Here's how the part is built. I have some questions about the finished solid (model axes, mm). Face numbers are marked on the shaded views. Give positions to 0.01 mm unless a question says otherwise; leave off trailing zeros. Write each loop counter-clockwise with the first axis right and the second up, starting at its lowest first coordinate (ties: lowest second). Pieces come first, ordered by that corner, then holes. Notation, with made-up numbers: (23, 53) - (48, 53) arc R26 cw to (48, 92) - close; hole circle Ø3 at (0.25, 10). An arc over 180 degrees is marked (long way). One line per item, written item: value. Start each with the question number.
1) Imagine slicing it at C-C on x = -8.5. Write out the boundary of the cut face in (y, z) (1 decimal), plus the area to 3 significant figures.
2) Imagine slicing it at D-D on z = -12.75. Write out the boundary of the cut face in (x, y).
3) Please list where these lines run through material, in increasing order: L1, parallel to Z at x = -2, y = -1; L2, parallel to Z at x = -9.75, y = -0.5 (1 decimal); L3, parallel to X at y = -1.1, z = -22. Write a range as [from, to].
4) We'd pull the mould along X, two halves only. Please class the marked faces 1 and 2: +X half, -X half, draft (parallel to the pull), parting line (faces both ways), or undercut.
5) Imagine slicing it at A-A on z = -18.5. Write out the boundary of the cut face in (x, y).
6) I'm going to push flat-ended pins straight in: P1, Ø0.8, axis at x = -8.5, y = -1.5, coming from the -Z side; P2, Ø5, axis at x = -7.5, z = -10, coming from the -Y side. Where does each tip first touch, or does it pass through?
Autodesk Inventor part; units mm, degrees
ref_plane "YZ Plane" through (0, 0, 0) normal (1, 0, 0) x (0, 1, 0)
ref_plane "XZ Plane" through (0, 0, 0) normal (0, 1, 0) x (-1, 0, 0)
ref_plane "XY Plane" through (0, 0, 0) normal (0, 0, 1) x (1, 0, 0)
sketch "Sketch1" plane through (0, 0, 0) normal (0, 1, 0) x (-1, 0, 0)
  line L0 (0, 0) -> (19.05, 0)
  line L1 (19.05, 0) -> (19.05, -24.003)
  line L2 (19.05, -24.003) -> (0, -24.003)
  line L3 (0, -24.003) -> (0, 0)
  dimension "d0" = 24.003
  dimension "d1" = 19.05
extrude "Extrusion1" add sketch "Sketch1" against normal blind 0.7937
fillet "Fillet1" radius 0.508 4 edges at (0, -0.3969, 0) (-19.05, -0.3969, 0) (0, -0.3969, -24.003) (-19.05, -0.3969, -24.003)
sketch "Sketch2" plane through (0, -0.7937, 0) normal (0, -1, 0) x (1, 0, 0)
  line L0 (-18.542, -24.003) -> (-0.508, -24.003)
  line L1 (0, -23.495) -> (0, -0.508)
  line L2 (-0.508, 0) -> (-18.542, 0)
  line L3 (-19.05, -0.508) -> (-19.05, -23.495)
  line L4 (-0.4572, -0.4572) -> (-18.5928, -0.4572)
  line L5 (-18.5928, -0.4572) -> (-18.5928, -23.5458)
  line L6 (-18.5928, -23.5458) -> (-0.4572, -23.5458)
  line L7 (-0.4572, -23.5458) -> (-0.4572, -0.4572)
  line L8 (-1.143, -1.143) -> (-17.907, -1.143)
  line L9 (-17.907, -1.143) -> (-17.907, -22.86)
  line L10 (-17.907, -22.86) -> (-1.143, -22.86)
  line L11 (-1.143, -22.86) -> (-1.143, -1.143)
  arc A0 (-19.05, -23.495) -> (-18.542, -24.003) centre (-18.542, -23.495) ccw
  arc A1 (-0.508, -24.003) -> (0, -23.495) centre (-0.508, -23.495) ccw
  arc A2 (0, -0.508) -> (-0.508, 0) centre (-0.508, -0.508) ccw
  arc A3 (-18.542, 0) -> (-19.05, -0.508) centre (-18.542, -0.508) ccw
  point P0 (0, 0)
  dimension "d5" = 0.4572
  dimension "d6" = 0.4572
  dimension "d7" = 0.4572
  dimension "d8" = 0.4572
  dimension "d9" = 1.143
  dimension "d10" = 1.143
  dimension "d11" = 1.143
  dimension "d12" = 1.143
extrude "Extrusion2" add sketch "Sketch2" along normal blind 0.7366 contours L7 L6 L5 L4
sketch "Sketch3" plane through (0, 0, 0) normal (0, 1, 0) x (1, 0, 0)
  arc A0 (-18.542, 24.003) -> (-19.05, 23.495) centre (-18.542, 23.495) ccw
  line L0 (-19.05, 23.495) -> (-19.05, 0.508)
  arc A1 (-19.05, 0.508) -> (-18.542, 0) centre (-18.542, 0.508) ccw
  line L1 (-18.542, 0) -> (-0.508, 0)
  arc A2 (-0.508, 0) -> (0, 0.508) centre (-0.508, 0.508) ccw
  line L2 (0, 0.508) -> (0, 23.495)
  arc A3 (0, 23.495) -> (-0.508, 24.003) centre (-0.508, 23.495) ccw
  line L3 (-0.508, 24.003) -> (-18.542, 24.003)
  line L4 (-11.1125, 19.685) -> (-7.9375, 19.685)
  line L5 (-7.9375, 19.685) -> (-7.9375, 14.9225)
  line L6 (-7.9375, 14.9225) -> (-11.1125, 14.9225)
  line L7 (-11.1125, 14.9225) -> (-11.1125, 19.685)
  point P0 (0, 0)
  dimension "d15" = 3.175
  dimension "d16" = 4.7625
  dimension "d17" = 19.05
  dimension "d18" = 7.9375
  dimension "d19" = 7.9375
  dimension "d20" = 4.318
extrude "Extrusion3" cut sketch "Sketch3" against normal blind 3.9116 contours L4 L5 L6 L7
fillet "Fillet2" radius 0.254 4 edges at (-11.1125, -0.3969, -19.685) (-7.9375, -0.3969, -19.685) (-7.9375, -0.3969, -14.9225) (-11.1125, -0.3969, -14.9225)
properties part number "Light Sensor Cover V1_3DPrint"
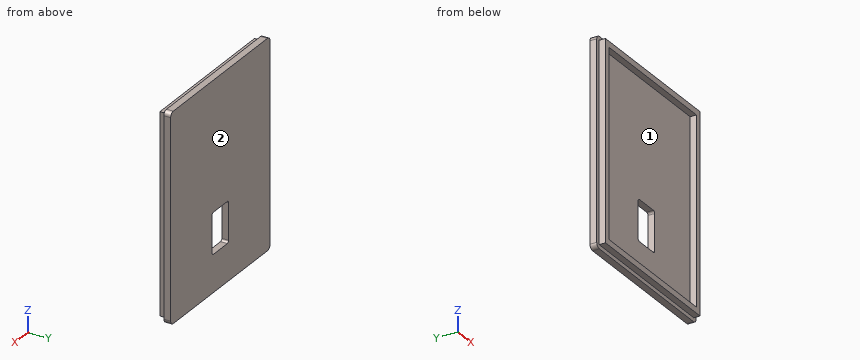
Numbers:
1. outline: (-1.5, -23.5) - (-0.8, -23.5) - (-0.8, -24) - (0, -24) - (0, -19.7) - (-0.8, -19.7) - (-0.8, -22.9) - (-1.5, -22.9) - close; (-1.5, -1.1) - (-0.8, -1.1) - (-0.8, -14.9) - (0, -14.9) - (0, 0) - (-0.8, 0) - (-0.8, -0.5) - (-1.5, -0.5) - close
1. area: 16.3 mm^2
2. outline: (-19.05, -0.79) - (-18.59, -0.79) - (-18.59, -1.53) - (-17.91, -1.53) - (-17.91, -0.79) - (-1.14, -0.79) - (-1.14, -1.53) - (-0.46, -1.53) - (-0.46, -0.79) - (0, -0.79) - (0, 0) - (-19.05, 0) - close
3. L1: [-23.55, -22.86], [-1.14, -0.46]
3. L2: [-24, -19.7], [-14.9, 0]
3. L3: [-18.59, -17.91], [-1.14, -0.46]
4. face 1: undercut
4. face 2: draft
5. outline: (-19.05, -0.79) - (-18.59, -0.79) - (-18.59, -1.53) - (-17.91, -1.53) - (-17.91, -0.79) - (-11.11, -0.79) - (-11.11, 0) - (-19.05, 0) - close; (-7.94, -0.79) - (-1.14, -0.79) - (-1.14, -1.53) - (-0.46, -1.53) - (-0.46, -0.79) - (0, -0.79) - (0, 0) - (-7.94, 0) - close
6. P1: z = -23.55
6. P2: y = -0.79
